Verification items for this drawing (mm, ordinates from the low corner). A direction names the side the tool comes from. Round coordinates to 2 decimals unless told otherwise and drop trailing zeros. Loops run counter-clockwise (first coordinate to the right, second up) from the corner with the lowest first, then second, coordinate; pieces in that order, holes last. Notation, with made-up numbers: M 81,-18 L 117,-18 A20 cw 117,-7 Z; hole C -25.5,-11 d2. An arc over 180 degrees is marked long. One line per item, written item: value.
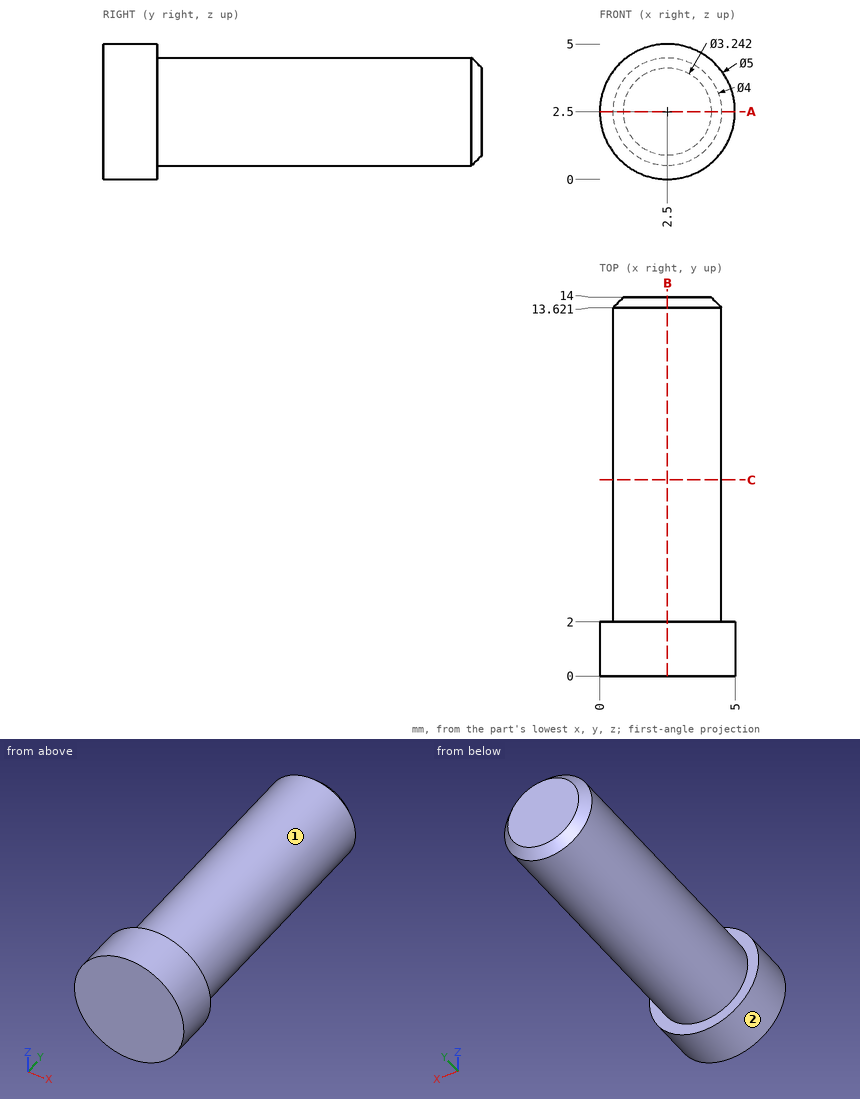
(1) Tool access check on the marked faces 1 and 2. Record the directions out of +Z, -Z, +X, -X, +Y, -Y that give a thin tool (end or side, any length) a straight path to the whole face; none if there is none.
Completed:
face 1: +Y
face 2: +Y, -Y
(2) Thickness scan on L1, parallel to Y at x = 1.85, z = 0.3; L2, parallel to X at y = 1, z = 1; L3, parallel to Z at x = 1.4, y = 2.5. Record the ranges inside material, lowest first. Write a range as from..to.
Completed:
L1: y = 0..2
L2: x = 0.5..4.5
L3: z = 0.83..4.17
(3) Sectioned sample at C-C on y = 7.25. Enter the section's corners in (x, z), and give its area (3 significant figures).
Completed:
outline: C 2.5,2.5 d4
area: 12.6 mm^2
(4) Sectioned sample at A-A on z = 2.5. Enter the section's corners in (x, y), and give its area (3 significant figures).
Completed:
outline: M 0,0 L 5,0 L 5,2 L 4.5,2 L 4.5,13.62 L 4.12,14 L 0.88,14 L 0.5,13.62 L 0.5,2 L 0,2 Z
area: 57.9 mm^2
(5) Depth check by flat-ended pin: pin 1 Ø1.5 at (y, z) = (5.5, 1.5) entering from -X. Enter the tip coordinate at first touch or a pass-through.
Completed:
pin 1: stops at x = 0.52
(6) Sectioned sample at B-B on x = 2.5. Enter the section's corners in (y, z), and give its area (3 significant figures).
Completed:
outline: M 0,0 L 2,0 L 2,0.5 L 13.62,0.5 L 14,0.88 L 14,4.12 L 13.62,4.5 L 2,4.5 L 2,5 L 0,5 Z
area: 57.9 mm^2
